from build123d import *

# Parameters (mm, degrees)
ESQUISSE1_W             = 11.5
ESQUISSE1_H             = 4.5
ESQUISSE1_W_2           = 18.5
ESQUISSE1_W_3           = 4
ESQUISSE1_H_2           = 14
BOSS_EXTRU_1_DEPTH      = 3
BOSS_EXTRU_2_DEPTH      = 3
ESQUISSE3_R             = 2
ESQUISSE3_R_2           = 0.5
BOSS_EXTRU_3_DEPTH      = 22.5
BOSS_EXTRU_4_START      = 1
ESQUISSE4_R             = 5
BOSS_EXTRU_4_DEPTH      = 1
ESQUISSE5_R             = 1.75
BOSS_EXTRU_5_DEPTH      = 3
ESQUISSE6_R             = 0.5
ENL_V_MAT_EXTRU_1_DEPTH = 7
ESQUISSE8_W             = 1.5
ESQUISSE8_H             = 4
BOSS_EXTRU_7_DEPTH      = 8
BOSS_EXTRU_8_DEPTH      = 4
BOSS_EXTRU_6_DEPTH      = 3
ESQUISSE10_W            = 4
ESQUISSE10_H            = 1.5
BOSS_EXTRU_9_DEPTH      = 14
BOSS_EXTRU_11_DEPTH     = 4
BOSS_EXTRU_12_DEPTH     = 4
BOSS_EXTRU_13_DEPTH     = 4
BOSS_EXTRU_14_DEPTH     = 4


with BuildPart() as part:
    # Esquisse1 → Boss.-Extru.1 (new body)
    with BuildSketch(Plane.XY):
        Polygon((-44, 32), (-44, 28), (-37.75, 28), (-37.75, 4), (-44, 4), (-44, 0), (0, 0), (0, 32), align=None)
        with Locations((-27, 25.75)):
            Rectangle(ESQUISSE1_W, ESQUISSE1_H, mode=Mode.SUBTRACT)
        with Locations((-23.5, 6.25)):
            Rectangle(ESQUISSE1_W_2, ESQUISSE1_H, mode=Mode.SUBTRACT)
        with Locations((-5, 16)):
            Rectangle(ESQUISSE1_W_3, ESQUISSE1_H_2, mode=Mode.SUBTRACT)
    boss_extru_1 = extrude(amount=BOSS_EXTRU_1_DEPTH)

    # Esquisse2 → Boss.-Extru.2 (add)
    with BuildSketch(Plane(origin=(0, 0, 0), x_dir=(0, 0, -1), z_dir=(1, 0, 0))):
        with BuildLine():
            Line((0, 32), (11.822414385, 32.42016324))
            ThreePointArc((11.822414385, 32.42016324), (16.109871823, 30.270940346), (16.616008757, 25.501739602))
            Line((16.616008757, 25.501739602), (6.256300568, 0.61568434))
            ThreePointArc((6.256300568, 0.61568434), (5.887934081, 0.168039767), (5.333098817, 0))
            Line((5.333098817, 0), (0, 0))
            Line((0, 0), (0, 32))
        make_face()
    boss_extru_2 = extrude(amount=-BOSS_EXTRU_2_DEPTH)

    # Esquisse3 → Boss.-Extru.3 (add)
    with BuildSketch(Plane(origin=(0, 0, 0), x_dir=(-1, 0, 0), z_dir=(0, 0, -1))):
        with Locations((19.25, 27)):
            Circle(ESQUISSE3_R)
        with Locations((19.25, 27)):
            Circle(ESQUISSE3_R_2, mode=Mode.SUBTRACT)
    boss_extru_3 = extrude(amount=BOSS_EXTRU_3_DEPTH)

    # Esquisse4 → Boss.-Extru.4 (add)
    with BuildSketch(Plane(origin=(0, 0, 0), x_dir=(0, 0, -1), z_dir=(1, 0, 0)).offset(BOSS_EXTRU_4_START)):
        with Locations((12, 27.4233179)):
            Circle(ESQUISSE4_R)
    boss_extru_4 = extrude(amount=-BOSS_EXTRU_4_DEPTH)

    # Esquisse5 → Boss.-Extru.5 (add)
    with BuildSketch(Plane(origin=(1, 0, 0), x_dir=(0, 0, -1), z_dir=(1, 0, 0))):
        with Locations((12, 27.4233179)):
            Circle(ESQUISSE5_R)
    boss_extru_5 = extrude(amount=BOSS_EXTRU_5_DEPTH)

    # Esquisse6 → Enlèv. mat.-Extru.1 (cut)
    with BuildSketch(Plane(origin=(4, 0, 0), x_dir=(0, 0, -1), z_dir=(1, 0, 0))):
        with Locations((12, 27.4233179)):
            Circle(ESQUISSE6_R)
    enl_v_mat_extru_1 = extrude(amount=-ENL_V_MAT_EXTRU_1_DEPTH, mode=Mode.SUBTRACT)

    # Esquisse8 → Boss.-Extru.7 (add)
    with BuildSketch(Plane(origin=(0, 0, 0), x_dir=(-1, 0, 0), z_dir=(0, 0, -1))):
        with Locations((37, 16)):
            Rectangle(ESQUISSE8_W, ESQUISSE8_H)
    boss_extru_7 = extrude(amount=BOSS_EXTRU_7_DEPTH)

    # Esquisse9 → Boss.-Extru.8 (add)
    with BuildSketch(Plane.XZ.offset(-14)):
        Polygon((-37.75, -8), (-38.75, -7), (-37.75, -7), align=None)
    boss_extru_8 = extrude(amount=-BOSS_EXTRU_8_DEPTH)

    # Symétrie1: Boss.-Extru.1, Boss.-Extru.2, Boss.-Extru.3, Boss.-Extru.4, Boss.-Extru.5, Enlèv. mat.-Extru.1, Boss.-Extru.7, Boss.-Extru.8 across plane
    add(boss_extru_1.mirror(Plane(origin=(-44, 32, 3), x_dir=(0, 0, 1), z_dir=(1, 0, 0))))
    add(boss_extru_2.mirror(Plane(origin=(-44, 32, 3), x_dir=(0, 0, 1), z_dir=(1, 0, 0))))
    add(boss_extru_3.mirror(Plane(origin=(-44, 32, 3), x_dir=(0, 0, 1), z_dir=(1, 0, 0))))
    add(boss_extru_4.mirror(Plane(origin=(-44, 32, 3), x_dir=(0, 0, 1), z_dir=(1, 0, 0))))
    add(boss_extru_5.mirror(Plane(origin=(-44, 32, 3), x_dir=(0, 0, 1), z_dir=(1, 0, 0))))
    add(enl_v_mat_extru_1.mirror(Plane(origin=(-44, 32, 3), x_dir=(0, 0, 1), z_dir=(1, 0, 0))), mode=Mode.SUBTRACT)
    add(boss_extru_7.mirror(Plane(origin=(-44, 32, 3), x_dir=(0, 0, 1), z_dir=(1, 0, 0))))
    add(boss_extru_8.mirror(Plane(origin=(-44, 32, 3), x_dir=(0, 0, 1), z_dir=(1, 0, 0))))

    # Esquisse7 → Boss.-Extru.6 (add)
    with BuildSketch(Plane(origin=(0, 0, 0), x_dir=(-1, 0, 0), z_dir=(0, 0, -1))):
        with BuildLine():
            Line((35.391133561, 30.087968026), (52.608866439, 30.087968026))
            ThreePointArc((52.608866439, 30.087968026), (44, 35), (35.391133561, 30.087968026))
        make_face()
    boss_extru_6 = extrude(amount=-BOSS_EXTRU_6_DEPTH)

    # Symétrie2: Boss.-Extru.6 across plane
    add(boss_extru_6.mirror(Plane(origin=(0, 16, 0), x_dir=(0, 0, 1), z_dir=(0, -1, 0))))

    # Esquisse10 → Boss.-Extru.9 (add)
    with BuildSketch(Plane.XY.offset(3)):
        with Locations((-29.75, 28.75)):
            Rectangle(ESQUISSE10_W, ESQUISSE10_H)
        with Locations((-24.25, 28.75)):
            Rectangle(ESQUISSE10_W, ESQUISSE10_H)
        with Locations((-29.75, 3.25)):
            Rectangle(ESQUISSE10_W, ESQUISSE10_H)
        with Locations((-17.25, 3.25)):
            Rectangle(ESQUISSE10_W, ESQUISSE10_H)
    extrude(amount=BOSS_EXTRU_9_DEPTH)

    # Esquisse11 → Boss.-Extru.11 (add)
    with BuildSketch(Plane(origin=(-15.25, 0, 0), x_dir=(0, 0, -1), z_dir=(1, 0, 0))):
        Polygon((-17, 4), (-17, 5), (-16, 4), align=None)
    extrude(amount=-BOSS_EXTRU_11_DEPTH)

    # Esquisse12 → Boss.-Extru.12 (add)
    with BuildSketch(Plane(origin=(-27.75, 0, 0), x_dir=(0, 0, -1), z_dir=(1, 0, 0))):
        Polygon((-17, 4), (-17, 5), (-16, 4), align=None)
    extrude(amount=-BOSS_EXTRU_12_DEPTH)

    # Esquisse13 → Boss.-Extru.13 (add)
    with BuildSketch(Plane(origin=(-22.25, 0, 0), x_dir=(0, 0, -1), z_dir=(1, 0, 0))):
        Polygon((-17, 28), (-17, 27), (-16, 28), align=None)
    extrude(amount=-BOSS_EXTRU_13_DEPTH)

    # Esquisse14 → Boss.-Extru.14 (add)
    with BuildSketch(Plane.ZY.offset(31.75)):
        Polygon((17, 28), (16, 28), (17, 27), align=None)
    extrude(amount=-BOSS_EXTRU_14_DEPTH)


solid = part.part
Work out the finished part from the listing and answer in its coordinate system (mm). A direction names the side the tool comes from. Coordinates: 2 decimals unless noted, no trailing zeros. Loops run counter-clockwise (first coordinate to the right, second up) from the corner with the lowest first, then second, coordinate; pieces in that order, holes last. Notation, with made-up numbers: (-9, -29) -> (15, -29) arc R15 cw to (15, 0) -> close; hole circle Ø7 at (-24, -27). An arc over 180 degrees is marked (long way). Write each question's results on one line, items separated by ' | '. Start each with the question number.
1) Find section A-A on z = 7.5. Determine the outline of the cut face in (x, y), then the cut area to 3 significant figures.
2) For faces 1 (the flat face through (-17, 2.5, 10)), 2 (the flat face through (-83, 9, 1)), 3 (the flat face through (-28, 28, 8)), determine the directions among +Z, -Z, +X, -X, +Y, -Y from which every point of the face is accessible in a straight line to the end or side of a thin tool.
3) The mould has two halves that part along X. Classify faces 4 (the flat face through (-83, 23, 1)), 5 (the flat face through (-31.75, 3, 10)), 6 (the flat face through (-30, 28, 17)): pulls with the +X half, pulls with the -X half, needs draft (parallel to the pull), parting line crosses it, or undercut.
4) Find section C-C on y = 15. Determine the outline of the cut face in (x, z), then the cut area to 3 significant figures.
5) Find section B-B on x = -30.5. Determine the outline of the cut face in (y, z).
6) Flat-ended cylindrical pins translate along their axes: P1, Ø4.5, axis at x = -30.5, z = 9.5, coming from the +Y side; P2, Ø3.5, axis at x = -27.5, z = 10, coming from the -Y side; P3, Ø1.5, axis at y = 5.5, z = 1, coming from the -X side. Find the tip coordinate at first contact, or state that the pin passes through.
7) Find section D-D on x = -46. Determine the outline of the cut face in (y, z), then the cut area to 3 significant figures.
8) Consider line 1 along X through (y, z) = (17, -4); line 2 along X through (y, z) = (24, -15); line 3 along X through (y, z) = (29, 14). Determine where each line is inside the solid, lowest interval first.
Response values:
1) outline: (-31.75, 2.5) -> (-27.75, 2.5) -> (-27.75, 4) -> (-31.75, 4) -> close; (-31.75, 28) -> (-27.75, 28) -> (-27.75, 29.5) -> (-31.75, 29.5) -> close; (-26.25, 28) -> (-22.25, 28) -> (-22.25, 29.5) -> (-26.25, 29.5) -> close; (-19.25, 2.5) -> (-15.25, 2.5) -> (-15.25, 4) -> (-19.25, 4) -> close | area: 24.0 mm^2
2) face 1: +Z, +X, -X, -Y | face 2: +Z, -Z | face 3: -Z
3) face 4: undercut | face 5: pulls with the -X half | face 6: needs draft
4) outline: (-88, -12.24) -> (-85, -12.24) -> (-85, 3) -> (-88, 3) -> close; (-81, 0) -> (-51.75, 0) -> (-51.75, -8) -> (-50.25, -8) -> (-49.25, -7) -> (-50.25, -7) -> (-50.25, 3) -> (-81, 3) -> close; (-38.75, -7) -> (-37.75, -8) -> (-36.25, -8) -> (-36.25, 0) -> (-7, 0) -> (-7, 3) -> (-37.75, 3) -> (-37.75, -7) -> close; (-3, -12.24) -> (0, -12.24) -> (0, 3) -> (-3, 3) -> close | area: 301 mm^2
5) outline: (0, 0) -> (4, 0) -> (4, 16) -> (5, 17) -> (2.5, 17) -> (2.5, 3) -> (0, 3) -> close; (8.5, 0) -> (23.5, 0) -> (23.5, 3) -> (8.5, 3) -> close; (27, 17) -> (28, 16) -> (28, 0) -> (32, 0) -> (32, 3) -> (29.5, 3) -> (29.5, 17) -> close
6) P1: stops at y = 29.5 | P2: stops at y = 2.5 | P3: stops at x = -88
7) outline: (-2.8, 0) -> (4, 0) -> (4, 3) -> (-2.8, 3) -> close; (28, 0) -> (34.8, 0) -> (34.8, 3) -> (28, 3) -> close | area: 40.8 mm^2
8) line 1: x = -88 to -85, -51.75 to -50.25, -37.75 to -36.25, -3 to 0 | line 2: x = -89 to -85, -3 to 1 | line 3: x = -31.75 to -27.75, -26.25 to -22.25
